Autodesk Inventor part; units mm, degrees
ref_plane "YZ Plane" through (0, 0, 0) normal (1, 0, 0) x (0, 1, 0)
ref_plane "XZ Plane" through (0, 0, 0) normal (0, 1, 0) x (-1, 0, 0)
ref_plane "XY Plane" through (0, 0, 0) normal (0, 0, 1) x (1, 0, 0)
sketch "Skizze1" plane through (0, 0, 0) normal (0, 0, 1) x (1, 0, 0)
  line L0 (-3.5, 3) -> (3.5, 3)
  line L1 (3.5, 3) -> (3.5, 0)
  line L2 (1.5, 0) -> (-1.5, 0)
  line L3 (-3.5, 0) -> (-3.5, 3)
  line L4 (-1.5, 0) -> (-1.5, -5)
  line L5 (-1.5, -5) -> (-3.5, -5)
  line L6 (-3.5, -5) -> (-3.5, 0)
  line L7 (1.5, -5) -> (3.5, -5)
  line L8 (3.5, -5) -> (3.5, 0)
  line L9 (1.5, 0) -> (1.5, -5)
  point P0 (0, 0)
  point P1 (0, 0)
  dimension "d1" = 5
  dimension "d2" = 7
  dimension "d3" = 2
  dimension "d7" = 0
  dimension "d8" = 5
  dimension "d9" = 2
  dimension "d24" = 3
extrude "Extrusion1" add sketch "Skizze1" along normal blind 3
sketch "Skizze2" plane through (0, 0, 3) normal (0, 0, 1) x (1, 0, 0)
  line L0 (3.5, -5) -> (3.5, 3)
  line L1 (-3.5, 3) -> (-3.5, -5)
  line L2 (-3.5, 0) -> (-1.5, 0)
  line L3 (1.5, 0) -> (3.5, 0)
  line L4 (-3.5, 1) -> (3.5, 1)
  line L5 (3.5, 0) -> (3.5, 1)
  line L6 (-3.5, 0) -> (-3.5, 1)
  line L7 (-1.5, 0) -> (1.5, 0)
  point P0 (0, 0)
  dimension "d20" = 1
extrude "Extrusion3" cut sketch "Skizze2" against normal blind 0.5
sketch "Skizze5" plane through (0, 0, 0) normal (0, 0, -1) x (-1, 0, 0)
  line L0 (1.5, 0) -> (-1.5, 0)
  line L1 (3.5, 3) -> (3.5, -5)
  line L2 (-3.5, -5) -> (-3.5, 3)
  line L3 (-3.5, 1) -> (3.5, 1)
  line L4 (3.5, 1) -> (3.5, 0)
  line L5 (3.5, 0) -> (-3.5, 0)
  line L6 (-3.5, 0) -> (-3.5, 1)
  point P0 (0, 0)
  point P1 (0, 0)
  dimension "d25" = 1
extrude "Extrusion5" cut sketch "Skizze5" against normal blind 0.5
properties part number "Leistende Kontakt" material "2.0401 CuZn39 Pb 3 (Messing)"
Build history of the part. All positions in model axes, mm. A direction names the side the tool comes from. Round coordinates to 2 decimals unless told otherwise and drop trailing zeros. Loops run counter-clockwise (first coordinate to the right, second up) from the corner with the lowest first, then second, coordinate; pieces in that order, holes last. Notation, with made-up numbers: (-4, 12.25) -> (25, 12.25) arc R27 cw to (25, 45.25) -> close; hole circle Ø8 at (-33.5, -23). An arc over 180 degrees is marked (long way). Use CSV: the item, a comma, the result in double quotes. Start each with the question number.
Q1. Flat gauge pins, fed straight in: pin 1 Ø0.6 at (x, z) = (-0.5, 0.5) entering from -Y; pin 2 Ø0.5 at (x, y) = (-1, 0.5) entering from +Z; pin 3 Ø0.8 at (x, y) = (-0.5, 0.5) entering from -Z. Where does each tip first touch, or does it go through?
Q2. Saw through at B-B on z = 0.75. Give the cut face in (x, y), and give its area (3 significant figures).
Q3. Saw through at D-D on z = 0.35. Give the cut face in (x, y), and give its area (3 significant figures).
Q4. Saw through at A-A on y = -1.25. Give the cut face in (x, z).
Q5. Mould opens along X. For faces 4 (the face through (-3, -2, 3)), 5 (the face through (-3.5, -1, 1)), 6 (the face through (0, 0, 1)) say: +X half, -X half, draft (parallel to the pull), parting line (faces both ways), or undercut.
Q6. Which spindle directions (+Z, -Z, +X, -X, +Y, -Y) get a long thin tool onto all of the face, cutting with end or side? Do faces 1 (the face through (0, 0.5, 2.5)), 2 (the face through (0, 0.5, 0.5)), 3 (the face through (1.5, -2, 1)). Say none if no direction does.
Q7. Saw through at C-C on x = 2.5. Give the cut face in (y, z).
Q8. Drill centre lines: L1, parallel to X at y = -1.5, z = 2.3; L2, parallel to Y at x = 3.25, z = 0.2; L3, parallel to Y at x = -1, z = 1. Where is each one in solid material? Low to high.
Solutions:
1,pin 1,"stops at y = 0"
1,pin 2,"stops at z = 2.5"
1,pin 3,"stops at z = 0.5"
2,outline,"(-3.5, -5) -> (-1.5, -5) -> (-1.5, 0) -> (1.5, 0) -> (1.5, -5) -> (3.5, -5) -> (3.5, 3) -> (-3.5, 3) -> close"
2,area,"41.0 mm^2"
3,outline,"(-3.5, -5) -> (-1.5, -5) -> (-1.5, 0) -> (-3.5, 0) -> close; (-3.5, 1) -> (3.5, 1) -> (3.5, 3) -> (-3.5, 3) -> close; (1.5, -5) -> (3.5, -5) -> (3.5, 0) -> (1.5, 0) -> close"
3,area,"34.0 mm^2"
4,outline,"(-3.5, 0) -> (-1.5, 0) -> (-1.5, 3) -> (-3.5, 3) -> close; (1.5, 0) -> (3.5, 0) -> (3.5, 3) -> (1.5, 3) -> close"
5,face 4,"draft"
5,face 5,"-X half"
5,face 6,"undercut"
6,face 1,"+Z, +X, -X"
6,face 2,"-Z, +X, -X"
6,face 3,"+Z, -Z, -Y"
7,outline,"(-5, 0) -> (0, 0) -> (0, 0.5) -> (1, 0.5) -> (1, 0) -> (3, 0) -> (3, 3) -> (1, 3) -> (1, 2.5) -> (0, 2.5) -> (0, 3) -> (-5, 3) -> close"
8,L1,"x = -3.5 to -1.5, 1.5 to 3.5"
8,L2,"y = -5 to 0, 1 to 3"
8,L3,"y = 0 to 3"
